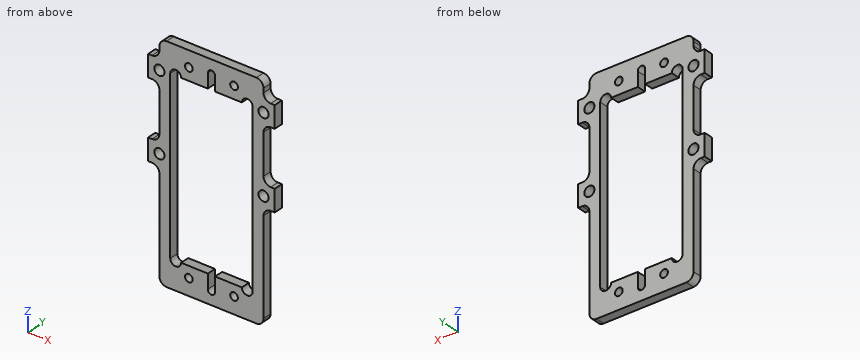
from build123d import *

# Parameters (mm, degrees)
SKETCH1_W                           = 28.956
SKETCH1_H                           = 59.69
BOSS_EXTRUDE1_DEPTH                 = 3.175
F_6_32_TAPPED_HOLE1_D               = 2.7051
F_6_32_TAPPED_HOLE1_DEPTH           = 3.175
F_9_64_0_14063_DIAMETER_HOLE1_D     = 3.572002
F_9_64_0_14063_DIAMETER_HOLE1_DEPTH = 3.175
FILLET1_R                           = 2.54
CUT_EXTRUDE1_REACH                  = 5.175
CUT_EXTRUDE2_REACH                  = 5.175


with BuildPart() as part:
    # Sketch1 → Boss-Extrude1 (new body)
    with BuildSketch(Plane(origin=(0, 0, 0), x_dir=(1, 0, 0), z_dir=(0, 1, 0))):
        Polygon((18.288, -23.8125), (18.288, -17.3228), (22.225, -17.3228), (22.225, -9.6647), (18.288, -9.6647), (18.288, 9.6647), (22.225, 9.6647), (22.225, 17.3228), (18.288, 17.3228), (18.288, 55.5625), (-18.288, 55.5625), (-18.288, 17.3228), (-22.225, 17.3228), (-22.225, 9.6647), (-18.288, 9.6647), (-18.288, -9.6647), (-22.225, -9.6647), (-22.225, -17.3228), (-18.288, -17.3228), (-18.288, -23.8125), align=None)
        with Locations((0, 15.954375)):
            Rectangle(SKETCH1_W, SKETCH1_H, mode=Mode.SUBTRACT)
    extrude(amount=BOSS_EXTRUDE1_DEPTH)

    # #6-32 Tapped Hole1
    with Locations(Plane.XZ):
        with Locations((-7.9375, 18.25625), (7.9375, 18.25625), (7.9375, -49.76495), (-7.9375, -49.76495)):
            Hole(F_6_32_TAPPED_HOLE1_D / 2, depth=F_6_32_TAPPED_HOLE1_DEPTH)

    # 9/64 (0.14063) Diameter Hole1
    with Locations(Plane.XZ):
        with Locations((18.288, -13.470384182), (18.288, 13.470384182), (-18.288, -13.470384182), (-18.288, 13.470384182)):
            Hole(F_9_64_0_14063_DIAMETER_HOLE1_D / 2, depth=F_9_64_0_14063_DIAMETER_HOLE1_DEPTH)

    # Fillet1
    fillet1_edges = [part.edges().sort_by_distance(p)[0] for p in [
        (18.288, 1.5875, 23.8125),
        (-18.288, 1.5875, 23.8125),
        (-18.288, 1.5875, 17.3228),
        (-18.288, 1.5875, 9.6647),
        (-18.288, 1.5875, -9.6647),
        (-18.288, 1.5875, -17.3228),
        (-18.288, 1.5875, -55.5625),
        (18.288, 1.5875, -55.5625),
        (18.288, 1.5875, -17.3228),
        (18.288, 1.5875, -9.6647),
        (18.288, 1.5875, 9.6647),
        (18.288, 1.5875, 17.3228),
    ]]
    fillet(fillet1_edges, radius=FILLET1_R)

    # Sketch7 → Cut-Extrude1 (cut, up to next)
    with BuildSketch(Plane(origin=(0, 3.175, 0), x_dir=(1, 0, 0), z_dir=(0, 1, 0)), mode=Mode.PRIVATE) as cut_extrude1_sk1:
        with BuildLine():
            Line((1.27, -13.890625), (1.27, -18.970625))
            ThreePointArc((1.27, -18.970625), (0, -20.240625), (-1.27, -18.970625))
            Line((-1.27, -18.970625), (-1.27, -13.890625))
            ThreePointArc((-1.27, -13.890625), (0, -12.620625), (1.27, -13.890625))
        make_face()
    cut_extrude1_tool1 = extrude(cut_extrude1_sk1.sketch, amount=-CUT_EXTRUDE1_REACH, mode=Mode.PRIVATE) & part.part
    add(cut_extrude1_tool1.solids().sort_by_distance((0, 3.175, 16.430625))[0], mode=Mode.SUBTRACT)
    # Sketch7 → Cut-Extrude1 (cut, up to next)
    with BuildSketch(Plane(origin=(0, 3.175, 0), x_dir=(1, 0, 0), z_dir=(0, 1, 0)), mode=Mode.PRIVATE) as cut_extrude1_sk2:
        with BuildLine():
            Line((-1.27, 45.799375), (-1.27, 50.879375))
            ThreePointArc((-1.27, 50.879375), (0, 52.149375), (1.27, 50.879375))
            Line((1.27, 50.879375), (1.27, 45.799375))
            ThreePointArc((1.27, 45.799375), (0, 44.529375), (-1.27, 45.799375))
        make_face()
    cut_extrude1_tool2 = extrude(cut_extrude1_sk2.sketch, amount=-CUT_EXTRUDE1_REACH, mode=Mode.PRIVATE) & part.part
    add(cut_extrude1_tool2.solids().sort_by_distance((0, 3.175, -48.339375))[0], mode=Mode.SUBTRACT)

    # Sketch8 → Cut-Extrude2 (cut, up to next)
    with BuildSketch(Plane(origin=(0, 3.175, 0), x_dir=(1, 0, 0), z_dir=(0, 1, 0)), mode=Mode.PRIVATE) as cut_extrude2_sk1:
        with BuildLine():
            Line((14.478, 45.799375), (10.668, 45.799375))
            ThreePointArc((10.668, 45.799375), (12.573, 47.704375), (14.478, 45.799375))
        make_face()
    cut_extrude2_tool1 = extrude(cut_extrude2_sk1.sketch, amount=-CUT_EXTRUDE2_REACH, mode=Mode.PRIVATE) & part.part
    add(cut_extrude2_tool1.solids().sort_by_distance((12.573, 3.175, -46.607882))[0], mode=Mode.SUBTRACT)
    # Sketch8 → Cut-Extrude2 (cut, up to next)
    with BuildSketch(Plane(origin=(0, 3.175, 0), x_dir=(1, 0, 0), z_dir=(0, 1, 0)), mode=Mode.PRIVATE) as cut_extrude2_sk2:
        with BuildLine():
            Line((-14.478, 45.799375), (-10.668, 45.799375))
            ThreePointArc((-10.668, 45.799375), (-12.573, 47.704375), (-14.478, 45.799375))
        make_face()
    cut_extrude2_tool2 = extrude(cut_extrude2_sk2.sketch, amount=-CUT_EXTRUDE2_REACH, mode=Mode.PRIVATE) & part.part
    add(cut_extrude2_tool2.solids().sort_by_distance((-12.573, 3.175, -46.607882))[0], mode=Mode.SUBTRACT)
    # Sketch8 → Cut-Extrude2 (cut, up to next)
    with BuildSketch(Plane(origin=(0, 3.175, 0), x_dir=(1, 0, 0), z_dir=(0, 1, 0)), mode=Mode.PRIVATE) as cut_extrude2_sk3:
        with BuildLine():
            Line((-14.478, -13.890625), (-10.668, -13.890625))
            ThreePointArc((-10.668, -13.890625), (-12.573, -15.795625), (-14.478, -13.890625))
        make_face()
    cut_extrude2_tool3 = extrude(cut_extrude2_sk3.sketch, amount=-CUT_EXTRUDE2_REACH, mode=Mode.PRIVATE) & part.part
    add(cut_extrude2_tool3.solids().sort_by_distance((-12.573, 3.175, 14.699132))[0], mode=Mode.SUBTRACT)
    # Sketch8 → Cut-Extrude2 (cut, up to next)
    with BuildSketch(Plane(origin=(0, 3.175, 0), x_dir=(1, 0, 0), z_dir=(0, 1, 0)), mode=Mode.PRIVATE) as cut_extrude2_sk4:
        with BuildLine():
            Line((10.668, -13.890625), (14.478, -13.890625))
            ThreePointArc((14.478, -13.890625), (12.573, -15.795625), (10.668, -13.890625))
        make_face()
    cut_extrude2_tool4 = extrude(cut_extrude2_sk4.sketch, amount=-CUT_EXTRUDE2_REACH, mode=Mode.PRIVATE) & part.part
    add(cut_extrude2_tool4.solids().sort_by_distance((12.573, 3.175, 14.699132))[0], mode=Mode.SUBTRACT)


solid = part.part
Can you work these out from the model? Positions are in its coordinate system, mm. Give positions to 0.01 mm unless a question says otherwise; leave off trailing zeros. Order: outer loops, then holes, each group sorted by start corner. A loop starts at its lowest first (then second) coordinate and runs counter-clockwise, first axis right, second up. Notation, with made-up numbers: M 34.25,-22 L 52.25,-22 A20 ccw 52.25,16 Z; hole C 85.5,38.25 d8. An arc over 180 degrees is marked long. One line per question, with ' | ' between items.
Item 1: Please list where these lines run through material, in increasing order: L1, parallel to X at y = 1.7, z = 13.5 (3 decimals); L2, parallel to X at y = 2.8, z = 2.5; L3, parallel to Z at x = -9.5, y = 1.4.
Answer block:
L1: x = -22.225 to -20.074, -16.502 to -14.478, 14.478 to 16.502, 20.074 to 22.225 | L2: x = -18.29 to -14.48, 14.48 to 18.29 | L3: z = -55.56 to -45.8, 13.89 to 23.81
Item 2: I'm going to push flat-ended pins straight in: pin 1 Ø0.7 at (y, z) = (1, 21) entering from +X; pin 2 Ø1.1 at (y, z) = (1, 21) entering from -X; pin 3 Ø1.1 at (x, y) = (-21.5, 1) entering from +Z. Where does each tip first touch, or does it pass through?
Answer block:
pin 1: stops at x = 18.29 | pin 2: stops at x = -18.29 | pin 3: stops at z = 17.32
Item 3: Suppose I cut it at B-B, the plane x = -3. Write out the boundary of the cut face in (y, z) (1 decimal), then the cut area to 3 significant figures.
Answer block:
outline: M 0,-55.6 L 3.2,-55.6 L 3.2,-45.8 L 0,-45.8 Z; M 0,13.9 L 3.2,13.9 L 3.2,23.8 L 0,23.8 Z | area: 62.5 mm2
Item 4: Suppose I cut it at C-C, the plane y = 1.3. Give the number of separate pieces and of enclosed holes in the cut face, then the cut area to 3 significant figures.
Answer block:
separate pieces: 1 | enclosed holes: 9 | area: 1,180 mm2
Item 5: Suppose I cut it at A-A, the plane z = -31. Write out the boundary of the cut face in (x, y) (3 decimals), then the cut area to 3 significant figures.
Answer block:
outline: M -18.288,0 L -14.478,0 L -14.478,3.175 L -18.288,3.175 Z; M 14.478,0 L 18.288,0 L 18.288,3.175 L 14.478,3.175 Z | area: 24.2 mm2
